Work out the finished part from the listing and answer in its coordinate system (mm). Face numbers are marked on the shaded views. A direction names the side the tool comes from. Coordinates: 2 decimals unless noted, no trailing zeros. Order: outer loops, then holes, each group sorted by start corner. A loop starts at its lowest first (then second) coordinate and runs counter-clockwise, first axis right, second up. Notation, with made-up numbers: (43.5, 74) -> (66.5, 74) arc R28 ccw to (66.5, 97) -> close; hole circle Ø3 at (8, 38.25). An arc over 180 degrees is marked (long way). Write item = value, one per line. Start each with the question number.
Q1. The part is cut by section B-B, the plane y = 0.5. Determine the outline of the cut face in (x, z).
Q2. Straight lines are drawn through the part: L1, parallel to Y at x = 0, z = 3.25; L2, parallel to Y at x = 0, z = 6.25; L3, parallel to Z at x = -3.5, y = 2.75. For each, find the intervals that lie inside material, in ascending order. Write a range as from..to.
Q3. For a pull along X with two mould halves and no side action, classify the marked faces 3, 4 and 5 as +X half, -X half, draft (parallel to the pull), parting line (faces both ways), or undercut.
Q4. A flat-ended cylindrical pin translates along its axis: pin 1 (1.5 mm diameter, centred on y = -2.5, z = 7, fed in from +X). Find the tip coordinate at first contact, or state that the pin passes through.
Q5. The part is cut by section A-A, the plane x = 0. Determine the outline of the cut face in (y, z), plus the area to 3 significant figures.
Q6. The part is cut by section C-C, the plane z = 2.5. Determine the outline of the cut face in (x, y).
Q7. Which of the six approach directions +Z, -Z, +X, -X, +Y, -Y give full straight-line access (tool end or side, diameter ignored) to the marked faces 1 and 2?
Q8. The part is cut by section D-D, the plane x = -3.75. Determine the outline of the cut face in (y, z), plus the area to 3 significant figures.
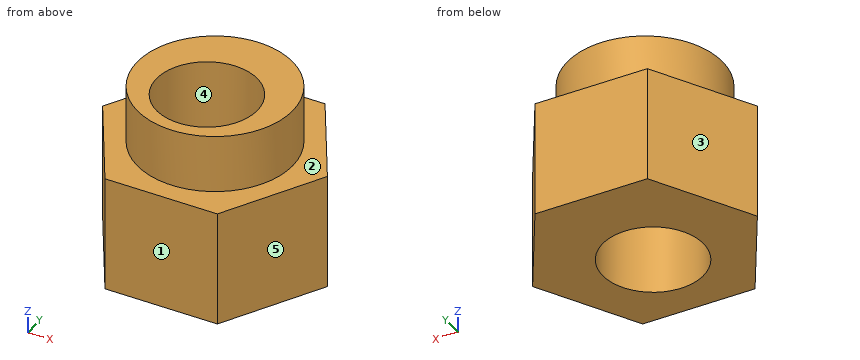
```python
from build123d import *

# Parameters (mm, degrees)
F2_R     = 4
F2_R_2   = 2.6
F3_DEPTH = 6
F4_DEPTH = 9


with BuildPart() as f3:
    # F2 (on Top) → F3 (new body)
    with BuildSketch(Plane.XY):
        Polygon((2.8867513459, 5), (-2.8867513459, 5), (-5.7735026919, 0), (-2.8867513459, -5), (2.8867513459, -5), (5.7735026919, 0), align=None)
        Circle(F2_R, mode=Mode.SUBTRACT)
        Circle(F2_R)
        with Locations((0, -0.75)):
            Circle(F2_R_2, mode=Mode.SUBTRACT)
    extrude(amount=F3_DEPTH)

    # F2 (on Top) → F4 (join)
    with BuildSketch(Plane.XY):
        Circle(F2_R)
        with Locations((0, -0.75)):
            Circle(F2_R_2, mode=Mode.SUBTRACT)
    extrude(amount=F4_DEPTH)


solid = f3.part
```
Model answer:
q1.outline = (-5.48, 0) -> (-2.28, 0) -> (-2.28, 9) -> (-3.97, 9) -> (-3.97, 6) -> (-5.48, 6) -> close; (2.28, 0) -> (5.48, 0) -> (5.48, 6) -> (3.97, 6) -> (3.97, 9) -> (2.28, 9) -> close
q2.L1 = -5..-3.35, 1.85..5
q2.L2 = -4..-3.35, 1.85..4
q2.L3 = 0..6
q3.face_3 = -X half
q3.face_4 = undercut
q3.face_5 = +X half
q4.pin_1 = 3.6
q5.outline = (-5, 0) -> (-3.35, 0) -> (-3.35, 9) -> (-4, 9) -> (-4, 6) -> (-5, 6) -> close; (1.85, 0) -> (5, 0) -> (5, 6) -> (4, 6) -> (4, 9) -> (1.85, 9) -> close
q5.area = 37.2 mm2
q6.outline = (-5.77, 0) -> (-2.89, -5) -> (2.89, -5) -> (5.77, 0) -> (2.89, 5) -> (-2.89, 5) -> close; hole circle Ø5.2 at (0, -0.75)
q7.face_1 = +Z, -Z, +X, -X, -Y
q7.face_2 = +Z
q8.outline = (-3.5, 0) -> (3.5, 0) -> (3.5, 6) -> (1.39, 6) -> (1.39, 9) -> (-1.39, 9) -> (-1.39, 6) -> (-3.5, 6) -> close
q8.area = 50.4 mm2
